```python
from build123d import *

# Parameters (mm, degrees)
BOSS_EXTRUDE1_DEPTH = 25
SKETCH2_R           = 2.2
CUT_EXTRUDE1_DEPTH  = 10
SKETCH4_W           = 21.020217786
SKETCH4_H           = 42.591039887
CUT_EXTRUDE2_DEPTH  = 14
SKETCH5_W           = 22.665717921
SKETCH5_H           = 57.45495938
CUT_EXTRUDE3_DEPTH  = 3
FILLET1_R           = 5
FILLET2_R           = 3
SKETCH6_R           = 4.5
CUT_EXTRUDE4_DEPTH  = 10
SKETCH8_W           = 42.21478983
SKETCH8_H           = 20.870122348
CUT_EXTRUDE5_DEPTH  = 21
SKETCH9_W           = 58.147470605
SKETCH9_H           = 20.870122348
CUT_EXTRUDE6_DEPTH  = 3
SKETCH10_R          = 2.2
CUT_EXTRUDE7_DEPTH  = 23


with BuildPart() as part:
    # Sketch1 → Boss-Extrude1 (new body)
    with BuildSketch(Plane.XY):
        Polygon((0, 100), (0, 0), (110, 0), (110, 100), (100, 100), (100, 10), (10, 10), (10, 100), align=None)
    extrude(amount=BOSS_EXTRUDE1_DEPTH)

    # Sketch2 → Cut-Extrude1 (cut)
    with BuildSketch(Plane.ZY):
        with Locations((7.5, 94.589613301)):
            Circle(SKETCH2_R)
        with Locations((17.5, 94.589613301)):
            Circle(SKETCH2_R)
        with Locations((7.5, 44.810386699)):
            Circle(SKETCH2_R)
        with Locations((17.5, 44.810386699)):
            Circle(SKETCH2_R)
    extrude(amount=-CUT_EXTRUDE1_DEPTH, mode=Mode.SUBTRACT)

    # Sketch4 → Cut-Extrude2 (cut)
    with BuildSketch(Plane(origin=(10, 0, 0), x_dir=(0, 0, -1), z_dir=(1, 0, 0))):
        with Locations((-12.458750101, 69.669580668)):
            Rectangle(SKETCH4_W, SKETCH4_H)
    extrude(amount=-CUT_EXTRUDE2_DEPTH, mode=Mode.SUBTRACT)

    # Sketch5 → Cut-Extrude3 (cut)
    with BuildSketch(Plane.ZY):
        with Locations((12.691576382, 69.375131892)):
            Rectangle(SKETCH5_W, SKETCH5_H)
    extrude(amount=-CUT_EXTRUDE3_DEPTH, mode=Mode.SUBTRACT)

    # Fillet1
    fillet1_edges = [part.edges().sort_by_distance(p)[0] for p in [
        (10, 10, 12.5),
        (100, 10, 12.5),
    ]]
    fillet(fillet1_edges, radius=FILLET1_R)

    # Fillet2
    fillet2_edges = [part.edges().sort_by_distance(p)[0] for p in [
        (5, 100, 0),
        (105, 100, 0),
        (110, 0, 12.5),
        (0, 0, 12.5),
        (5, 100, 25),
        (105, 100, 25),
    ]]
    fillet(fillet2_edges, radius=FILLET2_R)

    # Sketch6 → Cut-Extrude4 (cut)
    with BuildSketch(Plane(origin=(110, 0, 0), x_dir=(0, 0, -1), z_dir=(1, 0, 0))):
        with Locations((-12.5, 80)):
            Circle(SKETCH6_R)
    extrude(amount=-CUT_EXTRUDE4_DEPTH, mode=Mode.SUBTRACT)

    # Sketch8 → Cut-Extrude5 (cut)
    with BuildSketch(Plane.XZ):
        with Locations((44.714968541, 12.398762514)):
            Rectangle(SKETCH8_W, SKETCH8_H)
    extrude(amount=-CUT_EXTRUDE5_DEPTH, mode=Mode.SUBTRACT)

    # Sketch9 → Cut-Extrude6 (cut)
    with BuildSketch(Plane(origin=(0, 10, 0), x_dir=(1, 0, 0), z_dir=(0, 1, 0))):
        with Locations((44.434650342, -12.398762514)):
            Rectangle(SKETCH9_W, SKETCH9_H)
    extrude(amount=-CUT_EXTRUDE6_DEPTH, mode=Mode.SUBTRACT)

    # Sketch10 → Cut-Extrude7 (cut)
    with BuildSketch(Plane(origin=(0, 7, 0), x_dir=(1, 0, 0), z_dir=(0, 1, 0))):
        with Locations(Location((69.589613301, -7.5, 0), (0, 0, 270))):
            Circle(SKETCH10_R)
        with Locations(Location((69.589613301, -17.5, 0), (0, 0, 270))):
            Circle(SKETCH10_R)
        with Locations(Location((19.810386699, -7.5, 0), (0, 0, 270))):
            Circle(SKETCH10_R)
        with Locations(Location((19.810386699, -17.5, 0), (0, 0, 270))):
            Circle(SKETCH10_R)
    extrude(amount=-CUT_EXTRUDE7_DEPTH, mode=Mode.SUBTRACT)


solid = part.part
```
Check sheet for the modelled part. Datum: model origin and axes. Units: mm. A direction names the side the tool comes from. Give positions to 0.01 mm unless a question says otherwise; leave off trailing zeros. Order: outer loops, then holes, each group sorted by start corner. A loop starts at its lowest first (then second) coordinate and runs counter-clockwise, first axis right, second up. Notation, with made-up numbers: (83.5, -9.75) -> (141.5, -9.75) arc R20 ccw to (141.5, 10.25) -> close; hole circle Ø9 at (65, 44). An arc over 180 degrees is marked (long way). Use CSV: the item, a comma, the result in double quotes. Start each with the question number.
1) Sectioned sample at B-B, the plane x = 29. Record the boundary of the cut face in (y, z).
2) Material ranges on line 1 (Y direction, x = 7.5, z = 17.5); line 2 (X direction, y = 92, z = 23); line 3 (X direction, y = 27, z = 4.75), recorded low to high. Write a range as from..to.
3) Sectioned sample at A-A, the plane y = 16.5. Record the boundary of the cut face in (x, z).
4) Sectioned sample at C-C, the plane z = 12.5. Give the number of separate pieces and of enclosed holes in the cut face, plus the area to 3 significant figures.
5) Set-up check for faces 1 (the face through (65.822, 3, 12)), 2 (the face through (1, 40.648, 13)), 3 (the face through (70, 7, 12)), 4 (the face through (73, 10, 23)), 5 (the face through (5, 100, 12)): record each of +Z, -Z, +X, -X, +Y, -Y from which the full face is reachable in a straight line by a thin tool's end or side.
6) Go/stop test with flat-tipped pins: P1, Ø2.5, axis at x = 1.5, z = 17, coming from the -Y side; P2, Ø2.5, axis at x = 20, z = 16, coming from the +Y side; P3, Ø1, axis at x = 94, z = 13.5, coming from the +Y side; P4, Ø7, axis at y = 80, z = 12.5, coming from the -X side. Record where each tip stops, or that it passes through.
7) Mould release check, pull along Z, two halves, no side actions. Record for faces 6 (the face through (104.93, 99.1, 0.86)), 7 (the face through (6.451, 92.442, 17.023)), 8 (the face through (0.9, 0.86, 12.68)): released by +Z, released by -Z, zero draft, split by the parting line, or undercut.
Recorded:
1,outline,"(0, 0) -> (10, 0) -> (10, 1.96) -> (0, 1.96) -> close; (0, 22.83) -> (10, 22.83) -> (10, 25) -> (0, 25) -> close"
2,line 1,"0..42.61, 47.01..48.37, 90.97..92.39, 96.79..100"
2,line 2,"3..10, 100..110"
2,line 3,"0..10, 100..110"
3,outline,"(0, 0) -> (10, 0) -> (10, 25) -> (0, 25) -> close; (100, 0) -> (110, 0) -> (110, 25) -> (100, 25) -> close"
4,separate pieces,"4"
4,enclosed holes,"0"
4,area,"1,880 mm2"
5,face 1,"+Y, -Y"
5,face 2,"-X"
5,face 3,"+Y"
5,face 4,"+Z, -Z, +Y"
5,face 5,"+Z, -Z, +X, -X, +Y"
6,P1,"y = 0.01"
6,P2,"y = 7"
6,P3,"y = 10"
6,P4,"through"
7,face 6,"released by -Z"
7,face 7,"undercut"
7,face 8,"zero draft"
